Could you check a few things on this drawing? It's one solid part, dimensions in mm from its lowest x, y, z. A direction names the side the tool comes from. Give positions to 0.01 mm unless a question says otherwise; leave off trailing zeros. Loops run counter-clockwise (first coordinate to the right, second up) from the corner with the lowest first, then second, coordinate; pieces in that order, holes last. Notation, with made-up numbers: M 63,-36.5 L 84,-36.5 A17 ccw 84,-32.5 Z; hole C -33,52 d2. An arc over 180 degrees is marked long. Write each question's results on one line, items separated by ' | '. Start each with the question number.
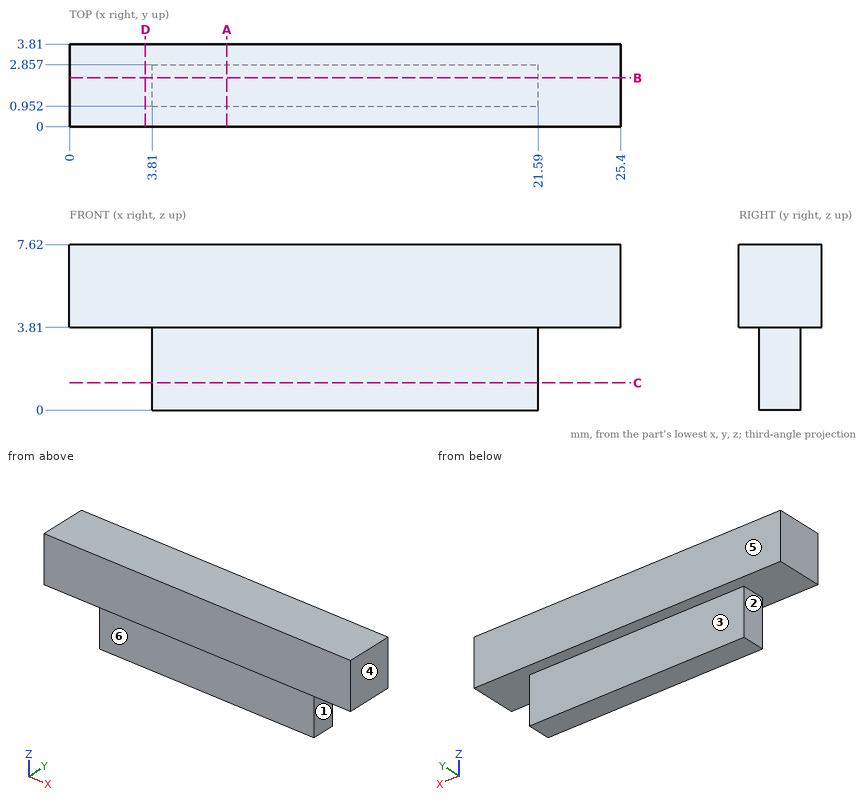
1) If we section it at D-D on x = 3.5: Write out the boundary of the cut face in (y, z), plus the area to 3 significant figures.
2) Please list where these lines run through material, in increasing order: line 1 (Z direction, x = 5, y = 0.45); line 2 (X direction, y = 1.8, z = 2); line 3 (Y direction, x = 17.5, z = 1.25). Write a range as from..to.
3) I'm going to push flat-ended pins straight in: P1, Ø1.9, axis at x = 9.5, z = 1.5, coming from the +Y side; P2, Ø1.5, axis at x = 7.5, y = 2.5, coming from the -Z side; P3, Ø1.1, axis at x = 10, z = 2.5, coming from the -Y side; P4, Ø0.6, axis at y = 2, z = 1, coming from the +X side. Where does each tip first touch, or does it pass through?
4) If we section it at C-C on z = 1.25: Write out the boundary of the cut face in (x, y).
5) Thinking about a two-plate mould opening in Y: for the marked faces 4, 5 and 6, which applies, pulls with the +Y half, pulls with the -Y half, needs draft (parallel to the pull), parting line crosses it, or undercut?
6) If we section it at A-A on x = 7.25: Write out the boundary of the cut face in (y, z).
7) If we section it at B-B on y = 2.25: Write out the boundary of the cut face in (x, z).
8) Which directions (+Z, -Z, +X, -X, +Y, -Y) give clear straight access to the entire face, cutting with the end or side of a thin tool? Please do the marked faces 1, 2 and 3.
Calculated:
1) outline: M 0,3.81 L 3.81,3.81 L 3.81,7.62 L 0,7.62 Z | area: 14.5 mm2
2) line 1: z = 3.81..7.62 | line 2: x = 3.81..21.59 | line 3: y = 0.95..2.86
3) P1: stops at y = 2.86 | P2: stops at z = 0 | P3: stops at y = 0.95 | P4: stops at x = 21.59
4) outline: M 3.81,0.95 L 21.59,0.95 L 21.59,2.86 L 3.81,2.86 Z
5) face 4: needs draft | face 5: pulls with the +Y half | face 6: pulls with the -Y half
6) outline: M 0,3.81 L 0.95,3.81 L 0.95,0 L 2.86,0 L 2.86,3.81 L 3.81,3.81 L 3.81,7.62 L 0,7.62 Z
7) outline: M 0,3.81 L 3.81,3.81 L 3.81,0 L 21.59,0 L 21.59,3.81 L 25.4,3.81 L 25.4,7.62 L 0,7.62 Z
8) face 1: -Z, +X, +Y, -Y | face 2: -Z, -X, +Y, -Y | face 3: -Z, +X, -X, +Y
